For this review, take the finished solid that the model builds, in its own axes (mm). A direction names the side the tool comes from. Round coordinates to 2 decimals unless told otherwise and drop trailing zeros. Order: outer loops, then holes, each group sorted by start corner. A loop starts at its lowest first (then second) coordinate and runs counter-clockwise, first axis right, second up. Notation, with made-up numbers: M 62,-35 L 115,-35 A19 ccw 115,2 Z; hole C 40.5,2 d6. An arc over 180 degrees is marked long. Use a Markdown table: item, result.
from build123d import *

# Parameters (mm, degrees)
SKETCH_1_R                   = 38
EXTRUDE_1_DEPTH              = 150
SKETCH_2_R                   = 10
EXTRUDE_2_DEPTH              = 80
SKETCH_3_R                   = 6
EXTRUDE_3_DEPTH              = 20
CUT_EXTRUDE_START            = 7.5
CUT_EXTRUDE_1_DEPTH          = 3
HOLE_WIZARD_M5_1_D           = 4.2
HOLE_WIZARD_M5_1_DEPTH       = 12.4
HOLE_WIZARD_M5_1_CSINK_D     = 5.05
HOLE_WIZARD_M5_1_CSINK_ANGLE = 90
HOLE_WIZARD_M5_1_TIP         = 1.2618073


with BuildPart() as part:
    # 草图1 → 凸台-拉伸1 (new, symmetric)
    with BuildSketch(Plane.XY):
        Circle(SKETCH_1_R)
    extrude(amount=EXTRUDE_1_DEPTH, both=True)

    # 草图2 → 凸台-拉伸2 (add)
    with BuildSketch(Plane.XY.offset(150)):
        Circle(SKETCH_2_R)
    extrude_2 = extrude(amount=EXTRUDE_2_DEPTH)

    # 镜向1: 凸台-拉伸2 across plane
    add(extrude_2.mirror(Plane.XY))

    # 草图3 → 凸台-拉伸3 (add)
    with BuildSketch(Plane.XY.offset(230)):
        Circle(SKETCH_3_R)
    extrude(amount=EXTRUDE_3_DEPTH)

    # 草图4 → 切除-拉伸1 (cut)
    with BuildSketch(Plane(origin=(0, 0, 0), x_dir=(1, 0, 0), z_dir=(0, 1, 0)).offset(CUT_EXTRUDE_START)):
        with BuildLine():
            Line((-2, -250), (-2, -235))
            ThreePointArc((-2, -235), (0, -233), (2, -235))
            Line((2, -235), (2, -250))
            ThreePointArc((2, -250), (0, -252), (-2, -250))
        make_face()
    extrude(amount=-CUT_EXTRUDE_1_DEPTH, mode=Mode.SUBTRACT)

    # M5 螺纹孔1
    with Locations(Plane.XY.offset(250)):
        with Locations((0, 0)):
            CounterSinkHole(HOLE_WIZARD_M5_1_D / 2, HOLE_WIZARD_M5_1_CSINK_D / 2, depth=HOLE_WIZARD_M5_1_DEPTH, counter_sink_angle=HOLE_WIZARD_M5_1_CSINK_ANGLE)
            with Locations((0, 0, -(HOLE_WIZARD_M5_1_DEPTH + HOLE_WIZARD_M5_1_TIP / 2))):  # 118° drill point
                Cone(0, HOLE_WIZARD_M5_1_D / 2, HOLE_WIZARD_M5_1_TIP, mode=Mode.SUBTRACT)


solid = part.part
Q1. Add section C-C (x = 20.5). Write out the cut boundary in (y, z).
Determined:
| item | result |
|---|---|
| outline | M -32,-150 L 32,-150 L 32,150 L -32,150 Z |
Q2. Clearance check with flat-ended pins moving along their axes: pin 1 (10 mm diameter, centred on x = 13.5, y = -15, fed in from -Z); pin 2 (10 mm diameter, centred on x = 18.5, y = -29, fed in from +Z); pin 3 (5.5 mm diameter, centred on x = 0, y = 0, fed in from +Z); pin 4 (2 mm diameter, centred on x = -19, z = -75, fed in from +Y). State where each tip first meets the part, or that it passes through.
Determined:
| item | result |
|---|---|
| pin 1 | stops at z = -150 |
| pin 2 | stops at z = 150 |
| pin 3 | stops at z = 250 |
| pin 4 | stops at y = 33.47 |
Q3. Add section D-D (z = 167.5). Write out the cut boundary in (x, y).
Determined:
| item | result |
|---|---|
| outline | C 0,0 d20 |
Q4. Machinability: for faces 1 (the flat face through (0, 0, -230)), 2 (the flat face through (8, -8, -150)), 3 (the cylindrical face through (-2.17, -9.76, 189.44)), which of the approach directions +Z, -Z, +X, -X, +Y, -Y give a long, thin tool a straight path to every point of the face, cutting with its end or side? Answer none if there is none.
Determined:
| item | result |
|---|---|
| face 1 | -Z, +X, -X, +Y, -Y |
| face 2 | -Z |
| face 3 | +Z |
Q5. Add section B-B (y = -17.5). Write out the cut boundary in (x, z).
Determined:
| item | result |
|---|---|
| outline | M -33.73,-150 L 33.73,-150 L 33.73,150 L -33.73,150 Z |
Q6. Add section A-A (z = -1). Write out the cut boundary in (x, y).
Determined:
| item | result |
|---|---|
| outline | C 0,0 d76 |
Q7. Wall thickness on line 1 along Y through (x, z) = (0, 246.25); line 2 along X through (y, z) = (0, 241.75); line 3 along Z through (x, y) = (20.5, -30.5): over which ranges is each line inside the solid? List them lowest first. Write a range as [from, to].
Determined:
| item | result |
|---|---|
| line 1 | y = [-6, -2.1], [2.1, 4.5] |
| line 2 | x = [-6, -2.1], [2.1, 6] |
| line 3 | z = [-150, 150] |
